Verification items for the finished model (mm, model axes). Face numbers are marked on the shaded views. A direction names the side the tool comes from. Give positions to 0.01 mm unless a question says otherwise; leave off trailing zeros. Order: outer loops, then holes, each group sorted by start corner. A loop starts at its lowest first (then second) coordinate and runs counter-clockwise, first axis right, second up. Notation, with made-up numbers: (85.25, -39) - (128.25, -39) arc R6 ccw to (128.25, -34) - close; hole circle Ø11 at (44, -3). An arc over 180 degrees is marked (long way). Answer as a JSON object with one key per item and string values.
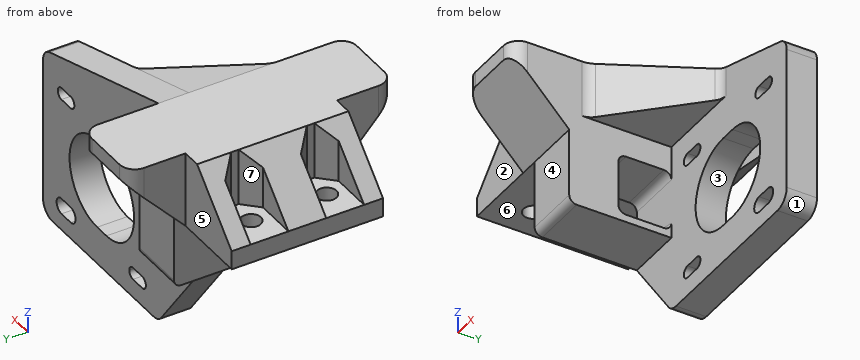
```python
from build123d import *

# Parameters (mm, degrees)
SKETCH1_W                = 40
SKETCH1_H                = 40
BOSS_EXTRUDE1_DEPTH      = 40
SKETCH2_W                = 25
SKETCH2_H                = 20
CUT_EXTRUDE1_DEPTH       = 40
CHAMFER1_SIZE            = 15
CUT_EXTRUDE2_DEPTH       = 15
CHAMFER2_SIZE            = 4
SKETCH4_R                = 2.6
CUT_EXTRUDE3_DEPTH       = 17
BOSS_EXTRUDE3_DEPTH      = 20
FILLET3_R                = 4
BOSS_EXTRUDE2_DEPTH      = 20
BOSS_EXTRUDE2_DEPTH_BACK = 25
SKETCH5_W                = 50
SKETCH5_H                = 8
CUT_EXTRUDE4_DEPTH       = 10
CHAMFER3_SIZE            = 15
CHAMFER3_SIZE_2          = 20
CHAMFER4_SIZE2           = 50
CHAMFER4_SIZE            = 15
FILLET5_START            = 26
FILLET5_DEPTH            = 10
FILLET6_R                = 2
CHAMFER5_START           = -40
CHAMFER5_DEPTH           = 40
CHAMFER5_START_2         = 2
CHAMFER5_2_DEPTH         = 25
SKETCH11_W               = 27.237482008
SKETCH11_H               = 25
CUT_EXTRUDE5_DEPTH       = 25
FILLET7_R                = 4
SKETCH16_W               = 14
SKETCH16_H               = 14
CUT_EXTRUDE6_DEPTH       = 43
CHAMFER6_SIZE            = 10
CHAMFER6_SIZE2           = 2
FILLET9_R                = 2


with BuildPart() as part:
    # Sketch1 → Boss-Extrude1 (new body)
    with BuildSketch(Plane(origin=(0, 0, 0), x_dir=(1, 0, 0), z_dir=(0, 1, 0))):
        with Locations((20, 20)):
            Rectangle(SKETCH1_W, SKETCH1_H)
    extrude(amount=BOSS_EXTRUDE1_DEPTH)

    # Sketch2 → Cut-Extrude1 (cut)
    with BuildSketch(Plane(origin=(0, 40, 0), x_dir=(1, 0, 0), z_dir=(0, 1, 0))):
        with Locations((12.5, 30)):
            Rectangle(SKETCH2_W, SKETCH2_H)
    extrude(amount=-CUT_EXTRUDE1_DEPTH, mode=Mode.SUBTRACT)

    # Chamfer1
    chamfer1_edges = [part.edges().sort_by_distance(p)[0] for p in [
        (0, 20, 0),
    ]]
    chamfer(chamfer1_edges, length=CHAMFER1_SIZE)

    # Sketch3 → Cut-Extrude2 (cut)
    with BuildSketch(Plane.XY):
        Polygon((0, 10), (0, 15), (15, 15), (15, 5), (0, 5), align=None)
        Polygon((0, 30), (0, 25), (15, 25), (15, 35), (0, 35), align=None)
    extrude(amount=-CUT_EXTRUDE2_DEPTH, mode=Mode.SUBTRACT)

    # Chamfer2
    chamfer2_edges = [part.edges().sort_by_distance(p)[0] for p in [
        (15, 35, -7.5),
        (15, 25, -7.5),
        (15, 15, -7.5),
        (15, 5, -7.5),
    ]]
    chamfer(chamfer2_edges, length=CHAMFER2_SIZE)

    # Sketch4 → Cut-Extrude3 (cut)
    with BuildSketch(Plane.XY.offset(-15)):
        with Locations((8, 30)):
            Circle(SKETCH4_R)
        with Locations((8, 10)):
            Circle(SKETCH4_R)
    extrude(amount=-CUT_EXTRUDE3_DEPTH, mode=Mode.SUBTRACT)

    # Sketch9 → Boss-Extrude3 (add)
    with BuildSketch(Plane(origin=(40, 0, 0), x_dir=(0, 0, -1), z_dir=(1, 0, 0))):
        Polygon((0, 40), (0, 55), (4, 55), (20, 40), align=None)
        Polygon((0, 0), (0, -15), (4, -15), (20, 0), align=None)
    extrude(amount=-BOSS_EXTRUDE3_DEPTH)

    # Fillet3
    fillet3_edges = [part.edges().sort_by_distance(p)[0] for p in [
        (20, 55, -2),
        (40, 55, -2),
        (20, -15, -2),
        (40, -15, -2),
    ]]
    fillet(fillet3_edges, radius=FILLET3_R)

    # Sketch5 → Boss-Extrude2 (add, two sides: drawn at the far end of the back side and taken through both)
    with BuildSketch(Plane(origin=(0, 0, -40), x_dir=(-1, 0, 0), z_dir=(0, 0, -1)).offset(-BOSS_EXTRUDE2_DEPTH_BACK)):
        with Locations((-65, 31)):
            Rectangle(SKETCH5_W, SKETCH5_H)
    extrude(amount=BOSS_EXTRUDE2_DEPTH + BOSS_EXTRUDE2_DEPTH_BACK)

    # Sketch10 → Cut-Extrude4 (cut)
    with BuildSketch(Plane(origin=(0, 27, 0), x_dir=(-1, 0, 0), z_dir=(0, -1, 0))):
        with BuildLine():
            ThreePointArc((-47, 51.9), (-45.4, 53.5), (-47, 55.1))
            Line((-47, 55.1), (-51, 55.1))
            ThreePointArc((-51, 55.1), (-52.13137085, 54.63137085), (-52.6, 53.5))
            ThreePointArc((-52.6, 53.5), (-52.13137085, 52.36862915), (-51, 51.9))
            Line((-51, 51.9), (-47, 51.9))
        make_face()
        with BuildLine():
            ThreePointArc((-47, 20.9), (-45.4, 22.5), (-47, 24.1))
            Line((-47, 24.1), (-51, 24.1))
            ThreePointArc((-51, 24.1), (-52.6, 22.5), (-51, 20.9))
            Line((-51, 20.9), (-47, 20.9))
        make_face()
        with BuildLine():
            ThreePointArc((-78, 20.9), (-76.4, 22.5), (-78, 24.1))
            Line((-78, 24.1), (-82, 24.1))
            ThreePointArc((-82, 24.1), (-83.6, 22.5), (-82, 20.9))
            Line((-82, 20.9), (-78, 20.9))
        make_face()
        with BuildLine():
            ThreePointArc((-66.5, 50), (-78.5, 38), (-66.5, 26))
            Line((-66.5, 26), (-62.5, 26))
            ThreePointArc((-62.5, 26), (-50.5, 38), (-62.5, 50))
            Line((-62.5, 50), (-66.5, 50))
        make_face()
        with BuildLine():
            ThreePointArc((-78, 51.4), (-75.9, 53.5), (-78, 55.6))
            Line((-78, 55.6), (-82, 55.6))
            ThreePointArc((-82, 55.6), (-84.1, 53.5), (-82, 51.4))
            Line((-82, 51.4), (-78, 51.4))
        make_face()
    extrude(amount=-CUT_EXTRUDE4_DEPTH, mode=Mode.SUBTRACT)

    # Chamfer3
    # the kernel refuses this chamfer: 20, 15 mm, written as the material it adds along each edge
    with BuildSketch(Plane(origin=(40, 27, -40), x_dir=(-1, 0, 0), z_dir=(0, 1, 0))) as chamfer3_piece_1:
        Polygon((CHAMFER3_SIZE, 0), (0, -CHAMFER3_SIZE_2), (0, 0), align=None)
    extrude(amount=8)

    # Chamfer4
    chamfer4_edges = [part.edges().sort_by_distance(p)[0] for p in [
        (40, 31, -15),
    ]]
    chamfer4_side = [part.faces().sort_by_distance(p)[0] for p in [
        (40, 31, -14.7),
    ]]
    chamfer(chamfer4_edges, length=CHAMFER4_SIZE - 0.0001, length2=CHAMFER4_SIZE2 - 0.0001, reference=chamfer4_side[0])  # a hair under: the kernel refuses the full size

    # Fillet5: read off the stored shape, not the designer's step
    # Fillet5 outline → Fillet5 (cut)
    with BuildSketch(Plane(origin=(0, 0, 0), x_dir=(1, 0, 0), z_dir=(0, 1, 0)).offset(FILLET5_START)):
        with BuildLine():
            Line((90, 15), (90, 17.976122604))
            ThreePointArc((90, 17.976122604), (89.209171713, 15.588400485), (87.149391542, 14.144817463))
            Line((87.149391542, 14.144817463), (90, 15))
        make_face()
        with BuildLine():
            ThreePointArc((38.8, 58.4), (40.211145618, 59.577708764), (42, 60))
            Line((42, 60), (40, 60))
            Line((40, 60), (38.8, 58.4))
        make_face()
        with BuildLine():
            ThreePointArc((86, 60), (88.828427125, 58.828427125), (90, 56))
            Line((90, 56), (90, 60))
            Line((90, 60), (86, 60))
        make_face()
    extrude(amount=FILLET5_DEPTH, mode=Mode.SUBTRACT)

    # Fillet6
    fillet6_edges = [part.edges().sort_by_distance(p)[0] for p in [
        (32.5, 40, -40),
        (32.5, 0, -40),
    ]]
    fillet(fillet6_edges, radius=FILLET6_R)

    # Chamfer5: read off the stored shape, not the designer's step
    # Chamfer5 outline → Chamfer5 (add)
    with BuildSketch(Plane.XY.offset(CHAMFER5_START)):
        Polygon((40, 5), (62, 27), (40, 27), align=None)
    extrude(amount=CHAMFER5_DEPTH)

    # Chamfer5 2 outline → Chamfer5 2 (cut)
    with BuildSketch(Plane(origin=(0, 0, 0), x_dir=(1, 0, 0), z_dir=(0, 1, 0)).offset(CHAMFER5_START_2)):
        with BuildLine():
            Line((51, 24.1), (47, 24.1))
            ThreePointArc((47, 24.1), (45.4, 22.5), (47, 20.9))
            Line((47, 20.9), (51, 20.9))
            ThreePointArc((51, 20.9), (52.6, 22.5), (51, 24.1))
        make_face()
        with BuildLine():
            ThreePointArc((50.667840434, 40), (53.33484861, 30.254033308), (62.5, 26))
            Line((62.5, 26), (64, 26))
            Line((64, 26), (64, 40))
            Line((64, 40), (50.667840434, 40))
        make_face()
        Polygon((64, 0), (64, 7.2), (40, 0), align=None)
    extrude(amount=CHAMFER5_2_DEPTH, mode=Mode.SUBTRACT)

    # Sketch11 → Cut-Extrude5 (cut)
    with BuildSketch(Plane(origin=(0, 0, -40), x_dir=(-1, 0, 0), z_dir=(0, 0, -1))):
        with Locations((-53.618741004, 14.5)):
            Rectangle(SKETCH11_W, SKETCH11_H)
    extrude(amount=-CUT_EXTRUDE5_DEPTH, mode=Mode.SUBTRACT)

    # Fillet7
    fillet7_edges = [part.edges().sort_by_distance(p)[0] for p in [
        (62, 27, -10.8000346),
        (40, 5, -7.5),
    ]]
    fillet(fillet7_edges, radius=FILLET7_R)

    # Sketch16 → Cut-Extrude6 (cut)
    with BuildSketch(Plane.ZY):
        with Locations((-29, 20)):
            Rectangle(SKETCH16_W, SKETCH16_H)
    extrude(amount=-CUT_EXTRUDE6_DEPTH, mode=Mode.SUBTRACT)

    # Chamfer6
    chamfer6_edges = [part.edges().sort_by_distance(p)[0] for p in [
        (40, 20, -36),
    ]]
    chamfer6_side = [part.faces().sort_by_distance(p)[0] for p in [
        (32.5, 20, -36),
    ]]
    chamfer(chamfer6_edges, length=CHAMFER6_SIZE, length2=CHAMFER6_SIZE2, reference=chamfer6_side[0])

    # Fillet9
    fillet9_edges = [part.edges().sort_by_distance(p)[0] for p in [
        (32.5, 13, -22),
        (32.5, 27, -22),
        (27.5, 27, -36),
        (27.5, 13, -36),
        (35, 13, -37),
        (35, 27, -37),
    ]]
    fillet(fillet9_edges, radius=FILLET9_R)


solid = part.part
```
(1) Material ranges on line 1 along Y through (x, z) = (8, -17.1); line 2 along Y through (x, z) = (50, -30); line 3 along X through (y, z) = (5, -19.5), recorded low to high. Write a range as [from, to].
Computed values:
{"line 1": "y = [0, 7.4], [12.6, 27.4], [32.6, 40]", "line 2": "y = [27, 35]", "line 3": "x = [0, 40]"}
(2) Access from +Z, -Z, +X, -X, +Y, -Y to the whole of each face (thin tool, end or side, straight path). Record for the marked faces 4, 5, 6 and 7.
Computed values:
{"face 4": "-Z, +X, -X, -Y", "face 5": "+Z, -Z, -X, +Y", "face 6": "-Z, -X, +Y, -Y", "face 7": "+Z, -X"}
(3) Section check A-A (y = 19). Record the cut outline in (x, z).
Computed values:
{"outline": "(0, -20) - (25, -20) - (25, -22) - (40, -22) - (40, -15) - (54, -15) - (54, -4.2) - (40, 0) - (15, 0) - (0, -15) - close; (25, -40) - (40, -40) - (40, -38) - (30, -36) - (25, -36) - close"}
(4) Release check for a two-part mould opening along Z. For the marked faces 1, 2 and 3 record: pulls with the +Z half, pulls with the -Z half, needs draft (parallel to the pull), parting line crosses it, or undercut.
Computed values:
{"face 1": "pulls with the -Z half", "face 2": "needs draft", "face 3": "undercut"}
(5) Section check B-B (x = 8). Record the cut outline in (y, z).
Computed values:
{"outline": "(0, -20) - (7.4, -20) - (7.4, -15) - (5, -15) - (5, -7) - (0, -7) - close; (12.6, -20) - (27.4, -20) - (27.4, -15) - (25, -15) - (25, -7) - (15, -7) - (15, -15) - (12.6, -15) - close; (32.6, -20) - (40, -20) - (40, -7) - (35, -7) - (35, -15) - (32.6, -15) - close"}
(6) Section check C-C (y = 36.5). Record the cut outline in (x, z).
Computed values:
{"outline": "(0, -20) - (25, -20) - (25, -40) - (40, -40) - (40, 0) - (15, 0) - (0, -15) - close"}
(7) Gauge pin test, flat ends, axial feed: pin 1 Ø8 at (x, z) = (27, -14) entering from -Y (3 decimals); pin 2 Ø16.5 at (x, y) = (30.5, 16) entering from -Z; pin 3 Ø10 at (y, z) = (-4.5, -10.5) entering from -X. Record the tip position at first contact, or that the pin passes through.
Computed values:
{"pin 1": "stops at y = -9.375", "pin 2": "stops at z = -40", "pin 3": "stops at x = 2.32"}
